Can you work these out from the model? Positions are in its coordinate system, mm. A direction names the side the tool comes from. Round coordinates to 2 decimals unless told otherwise and drop trailing zeros. Loops run counter-clockwise (first coordinate to the right, second up) from the corner with the lowest first, then second, coordinate; pieces in that order, holes last.
(1) I want a section at A-A on z = 64.5. Write out the boundary of the cut face in (x, y).
(2) I want a section at C-C on x = 107. Write out the boundary of the cut face in (y, z), plus the area to 3 significant figures.
(3) If I drill on line 1 along X through (y, z) = (36, 69.5); line 2 along X through (y, z) = (42.5, 14.5); line 3 along Z through (x, y) = (54.5, 55.5), over which ranges is the centre line in solid material (lowest first)?
(4) I want a section at D-D on y = 29. Write out the boundary of the cut face in (x, z).
(5) Which directions (+Z, -Z, +X, -X, +Y, -Y) give clear straight access to the entire face, cutting with the end or side of a thin tool? Please do faces 1 (the face through (65.42, 86.64, 23.72)), 2 (the face through (123.03, 53.22, 46.1)), 3 (the face through (2, 62, 24)), 4 (the face through (1.972, 86.113, 30.694)).
(6) I want a section at B-B on y = 96. Write out the boundary of the cut face in (x, z), plus the area to 3 significant figures.
(7) Will these pins go through, and if not, where does the flat tip stop? pin 1 Ø1.6 at (y, z) = (77.5, 19) entering from +X; pin 2 Ø5 at (x, y) = (7, 118) entering from +Z; pin 3 Ø3 at (x, y) = (63.5, 88) entering from +Z.
(8) Thinking about a two-plate mould opening in Z: for faces 5 (the face through (61, 101, 21.3)), 6 (the face through (2, 62, 44)), 7 (the face through (67.2, 45.2, 23.7)), 8 (the face through (62, 63, 0)), which applies, released by +Z, released by -Z, zero draft, split by the parting line, or undercut?
from build123d import *

# Parameters (mm, degrees)
SKIZZE1_W                       = 125
SKIZZE1_H                       = 125
AUFSATZ_LINEAR_AUSTRAGEN1_DEPTH = 2
SKIZZE2_W                       = 117
SKIZZE2_H                       = 117
AUFSATZ_LINEAR_AUSTRAGEN2_DEPTH = 2
SKIZZE3_R                       = 2
SCHNITT_LINEAR_AUSTRAGEN1_DEPTH = 32
AUFSATZ_LINEAR_AUSTRAGEN3_DEPTH = 40
SKIZZE8_R                       = 1
SCHNITT_LINEAR_AUSTRAGEN3_DEPTH = 40
SKIZZE9_R                       = 3.493135661
SCHNITT_LINEAR_AUSTRAGEN4_DEPTH = 20
SKIZZE10_W                      = 4
SKIZZE10_H                      = 125
AUFSATZ_LINEAR_AUSTRAGEN4_DEPTH = 70
SKIZZE11_R                      = 15.25
SKIZZE11_R_2                    = 1
SCHNITT_LINEAR_AUSTRAGEN5_DEPTH = 10
SKIZZE12_R                      = 15.25
SKIZZE12_R_2                    = 1
SKIZZE12_W                      = 20
SKIZZE12_H                      = 20
SCHNITT_LINEAR_AUSTRAGEN6_DEPTH = 12
SKIZZE13_R                      = 1
SCHNITT_LINEAR_AUSTRAGEN7_DEPTH = 10
SCHNITT_LINEAR_AUSTRAGEN8_DEPTH = 22.7


with BuildPart() as part:
    # Skizze1 → Aufsatz-Linear austragen1 (new body)
    with BuildSketch(Plane.XY):
        with Locations((62.5, 62.5)):
            Rectangle(SKIZZE1_W, SKIZZE1_H)
    extrude(amount=AUFSATZ_LINEAR_AUSTRAGEN1_DEPTH)

    # Skizze2 → Aufsatz-Linear austragen2 (add)
    with BuildSketch(Plane.XY.offset(2)):
        with Locations((62.5, 62.5)):
            Rectangle(SKIZZE2_W, SKIZZE2_H)
    extrude(amount=AUFSATZ_LINEAR_AUSTRAGEN2_DEPTH)

    # Skizze3 → Schnitt-Linear austragen1 (cut)
    with BuildSketch(Plane.XY.offset(4)):
        with Locations((7, 118)):
            Circle(SKIZZE3_R)
        with Locations((7, 7)):
            Circle(SKIZZE3_R)
        with Locations((118, 7)):
            Circle(SKIZZE3_R)
        with Locations((118, 118)):
            Circle(SKIZZE3_R)
    extrude(amount=-SCHNITT_LINEAR_AUSTRAGEN1_DEPTH, mode=Mode.SUBTRACT)

    # Skizze4 → Aufsatz-Linear austragen3 (add)
    with BuildSketch(Plane.XY.offset(4)):
        Polygon((62.595258591, 85.778313546), (68.333087126, 87.532543775), (59.561935985, 116.221686454), (53.824107449, 114.467456225), align=None)
        Polygon((54.200560001, 46.732563956), (73.26842417, 33.871127177), (76.623581591, 38.845352612), (57.555717422, 51.706789392), align=None)
    extrude(amount=AUFSATZ_LINEAR_AUSTRAGEN3_DEPTH)

    # Skizze8 → Schnitt-Linear austragen3 (cut)
    with BuildSketch(Plane(origin=(-27.403744567, 89.633609675, 0), x_dir=(0.9563047559630352, 0.2923717047227376, 0), z_dir=(-0.29237170472273766, 0.9563047559630353, 0))):
        with Locations(Location((87.939295251, -34, 0), (0, 0, 180))):
            Circle(SKIZZE8_R)
    extrude(amount=-SCHNITT_LINEAR_AUSTRAGEN3_DEPTH, mode=Mode.SUBTRACT)

    # Skizze9 → Schnitt-Linear austragen4 (cut)
    with BuildSketch(Plane(origin=(41.968333241, 62.220612777, 0), x_dir=(0.8290375725550413, -0.5591929034707476, 0), z_dir=(0.5591929034707476, 0.8290375725550413, 0))):
        with Locations(Location((30.301782569, -34, 0), (0, 0, 180))):
            Circle(SKIZZE9_R)
    extrude(amount=-SCHNITT_LINEAR_AUSTRAGEN4_DEPTH, mode=Mode.SUBTRACT)

    # Skizze10 → Aufsatz-Linear austragen4 (add)
    with BuildSketch(Plane.XY.offset(2)):
        with Locations((123, 62.5)):
            Rectangle(SKIZZE10_W, SKIZZE10_H)
        with Locations((2, 62.5)):
            Rectangle(SKIZZE10_W, SKIZZE10_H)
    extrude(amount=AUFSATZ_LINEAR_AUSTRAGEN4_DEPTH)

    # Skizze11 → Schnitt-Linear austragen5 (cut)
    with BuildSketch(Plane(origin=(125, 0, 0), x_dir=(0, 0, -1), z_dir=(1, 0, 0))):
        with Locations((-34, 62.5)):
            Circle(SKIZZE11_R)
        with Locations((-49, 47.5)):
            Circle(SKIZZE11_R_2)
        with Locations((-19, 47.5)):
            Circle(SKIZZE11_R_2)
        with Locations((-49, 77.5)):
            Circle(SKIZZE11_R_2)
        with Locations((-19, 77.5)):
            Circle(SKIZZE11_R_2)
    extrude(amount=-SCHNITT_LINEAR_AUSTRAGEN5_DEPTH, mode=Mode.SUBTRACT)

    # Skizze12 → Schnitt-Linear austragen6 (cut)
    with BuildSketch(Plane.ZY):
        with Locations((34, 101)):
            Circle(SKIZZE12_R)
        with Locations((19, 116)):
            Circle(SKIZZE12_R_2)
        with Locations((49, 116)):
            Circle(SKIZZE12_R_2)
        with Locations((49, 86)):
            Circle(SKIZZE12_R_2)
        with Locations((19, 86)):
            Circle(SKIZZE12_R_2)
        with Locations((19, 72.5)):
            Circle(SKIZZE12_R_2)
        with Locations((49, 72.5)):
            Circle(SKIZZE12_R_2)
        with Locations((49, 52.5)):
            Circle(SKIZZE12_R_2)
        with Locations((19, 52.5)):
            Circle(SKIZZE12_R_2)
        with Locations((34, 62.5)):
            Rectangle(SKIZZE12_W, SKIZZE12_H)
    extrude(amount=-SCHNITT_LINEAR_AUSTRAGEN6_DEPTH, mode=Mode.SUBTRACT)

    # Skizze13 → Schnitt-Linear austragen7 (cut)
    with BuildSketch(Plane.ZY):
        with Locations((24, 52.5)):
            Circle(SKIZZE13_R)
        with Locations((44, 52.5)):
            Circle(SKIZZE13_R)
        with Locations((24, 72.5)):
            Circle(SKIZZE13_R)
        with Locations((44, 72.5)):
            Circle(SKIZZE13_R)
    extrude(amount=-SCHNITT_LINEAR_AUSTRAGEN7_DEPTH, mode=Mode.SUBTRACT)

    # Skizze7 → Schnitt-Linear austragen8 (cut)
    with BuildSketch(Plane.XY.offset(44)):
        Polygon((54.49656237, 112.267955287), (60.234390906, 114.022185515), (67.660632206, 89.732044713), (61.92280367, 87.977814485), align=None)
    extrude(amount=-SCHNITT_LINEAR_AUSTRAGEN8_DEPTH, mode=Mode.SUBTRACT)


solid = part.part
Filled sheet:
1. outline: (0, 0) - (4, 0) - (4, 125) - (0, 125) - close; (121, 0) - (125, 0) - (125, 125) - (121, 125) - close
2. outline: (0, 0) - (125, 0) - (125, 2) - (121, 2) - (121, 4) - (4, 4) - (4, 2) - (0, 2) - close
2. area: 484 mm2
3. line 1: x = 0 to 4, 121 to 125
3. line 2: x = 0 to 4, 60.48 to 71.21, 121 to 125
3. line 3: z = 0 to 4
4. outline: (0, 0) - (125, 0) - (125, 72) - (121, 72) - (121, 4) - (4, 4) - (4, 72) - (0, 72) - close
5. face 1: +Z
5. face 2: +X
5. face 3: +X, -X
5. face 4: -X
6. outline: (0, 0) - (125, 0) - (125, 72) - (121, 72) - (121, 4) - (65.74, 4) - (65.74, 21.3) - (59.47, 21.3) - (59.47, 4) - (4, 4) - (4, 19.59) - (0, 19.59) - close; (0, 48.41) - (4, 48.41) - (4, 72) - (0, 72) - close
6. area: 1,040 mm2
7. pin 1: stops at x = 4
7. pin 2: stops at z = 4
7. pin 3: stops at z = 44
8. face 5: released by +Z
8. face 6: undercut
8. face 7: zero draft
8. face 8: released by -Z
